```python
from build123d import *

# Parameters (mm, degrees)
F0_R     = 21.2656768744
F0_R_2   = 25.5883994311
F0_R_3   = 15.3385974219
F0_W     = 29.6467319131
F0_H     = 12.3528018594
F1_DEPTH = 41.148
F3_DEPTH = 62.738
F4_W     = 45.1700200792
F4_H     = 28.5053551197
F5_DEPTH = 16.764


with BuildPart() as f1:
    # F0 (on Top) → F1 (new body)
    with BuildSketch(Plane.XY):
        Polygon((86.1493721604, -51.383343386), (86.1493721604, 51.383343386), (-86.1493721604, 51.383343386), (-86.1493721604, -39.0305415266), (-56.5026402473, -39.0305415266), (-56.5026402473, -51.383343386), align=None)
        with Locations((32.0047549903, -21.087879315)):
            Circle(F0_R, mode=Mode.SUBTRACT)
        with Locations((-33.9969657362, 17.5746399909)):
            Circle(F0_R_2, mode=Mode.SUBTRACT)
        with Locations((42.4747541547, 26.905214414)):
            Circle(F0_R_3, mode=Mode.SUBTRACT)
        with Locations((-71.3260062039, -45.2069424563)):
            Rectangle(F0_W, F0_H)
        Polygon((-86.1493721604, -51.383343386), (-86.1493721604, -39.0305415266), (-115.7961040735, -39.0305415266), (-115.7961040735, -63.7361452454), (-56.5026402473, -63.7361452454), (-56.5026402473, -51.383343386), align=None)
    extrude(amount=F1_DEPTH)

    # F2 (on face) → F3 (cut)
    with BuildSketch(Plane.XZ.offset(63.7361452454)):
        Polygon((-82.8842633783, 3.5929778848), (-72.3024426285, 26.3603644998), (-95.0698292435, 36.9421852496), (-105.6516499933, 14.1747986345), align=None)
    extrude(amount=-F3_DEPTH, mode=Mode.SUBTRACT)

    # F4 (on Top) → F5 (cut)
    with BuildSketch(Plane.XY):
        with Locations((-26.1654389324, -31.664095819)):
            Rectangle(F4_W, F4_H)
    extrude(amount=F5_DEPTH, mode=Mode.SUBTRACT)


solid = f1.part
```
Source: CAD feature listing. Evaluate the final solid. Frame: model axes, mm. A direction names the side the tool comes from. Give positions to 0.01 mm unless a question says otherwise; leave off trailing zeros. Order: outer loops, then holes, each group sorted by start corner. A loop starts at its lowest first (then second) coordinate and runs counter-clockwise, first axis right, second up.
(1) Access query for faces 1 (the face through (-56.503, -58, 20)), 2 (the face through (-104, -39.031, 20)), 3 (the face through (-26, -17.411, 8)), 4 (the face through (-80.997, -32.806, 30.401)). Directions: +Z, -Z, +X, -X, +Y, -Y. A direction counts if a zero-diameter tool reaches every point of the face in a straight line with its end or side. Return the directions, or none.
(2) Section query A-A (z = 19). Return the cut outline in (x, y), plus the area to 3 significant figures.
(3) Section query C-C (y = 9). Return the cut outline in (x, z).
(4) Material intervals for line 1 along X through (y, z) = (23.5, 17.5); line 2 along X through (y, z) = (20.5, 19); line 3 along X through (y, z) = (-25.5, 33), sorted ascending.
(5) Pull-direction query (Z, two-part tool) for faces 5 (the face through (-16, -5, 41.148)), 6 (the face through (-94.43, -46.75, 8.96)), 7 (the face through (-73, -63.736, 20)); classes: +Z half, -Z half, draft (parallel to the pull), parting line (faces both ways), or undercut.
(6) Section query D-D (x = -28.5). Return the cut outline in (y, z), plus the area to 3 significant figures.
(7) Contact query for flat-ended pins moving along their axis: P1, Ø15, axis at x = -80, z = 20.5, coming from the -Y side; P2, Ø5, axis at y = -26, z = 10.5, coming from the -X side; P3, Ø3, axis at y = 14, z = 16.5, coming from the -X side; P4, Ø5, axis at x = -31, z = 12, coming from the -Y side. Output: stop coordinate, or through.
(8) Section query B-B (x = 34). Return the cut outline in (y, z), plus the area to 3 significant figures.
Outcome:
1. face 1: +Z, -Z, +X, -Y
1. face 2: +Z, -Z, -X, +Y
1. face 3: -Z
1. face 4: -Y
2. outline: (-115.8, -63.74) - (-103.41, -63.74) - (-103.41, -39.03) - (-115.8, -39.03) - close; (-86.15, -1) - (-75.72, -1) - (-75.72, -63.74) - (-56.5, -63.74) - (-56.5, -51.38) - (86.15, -51.38) - (86.15, 51.38) - (-86.15, 51.38) - close; hole circle Ø51.18 at (-34, 17.57); hole circle Ø42.53 at (32, -21.09); hole circle Ø30.68 at (42.47, 26.91)
2. area: 13,500 mm2
3. outline: (-86.15, 0) - (-58.11, 0) - (-58.11, 41.15) - (-86.15, 41.15) - close; (-9.89, 0) - (86.15, 0) - (86.15, 41.15) - (-9.89, 41.15) - close
4. line 1: x = -86.15 to -58.89, -9.1 to 27.52, 57.43 to 86.15
4. line 2: x = -86.15 to -59.42, -8.58 to 28.54, 56.41 to 86.15
4. line 3: x = -86.15 to 11.2, 52.81 to 86.15
5. face 5: +Z half
5. face 6: undercut
5. face 7: draft
6. outline: (-51.38, 0) - (-45.92, 0) - (-45.92, 16.76) - (-17.41, 16.76) - (-17.41, 0) - (-7.42, 0) - (-7.42, 41.15) - (-51.38, 41.15) - close; (42.57, 0) - (51.38, 0) - (51.38, 41.15) - (42.57, 41.15) - close
6. area: 1,690 mm2
7. P1: stops at y = -63.74
7. P2: stops at x = -80.84
7. P3: stops at x = -86.15
7. P4: stops at y = -51.38
8. outline: (-51.38, 0) - (-42.26, 0) - (-42.26, 41.15) - (-51.38, 41.15) - close; (0.08, 0) - (14.12, 0) - (14.12, 41.15) - (0.08, 41.15) - close; (39.69, 0) - (51.38, 0) - (51.38, 41.15) - (39.69, 41.15) - close
8. area: 1,430 mm2
